Source: CAD feature listing. Evaluate the final solid. Frame: model axes, mm. Round coordinates to 2 decimals unless told otherwise and drop trailing zeros. Order: outer loops, then holes, each group sorted by start corner. A loop starts at its lowest first (then second) coordinate and runs counter-clockwise, first axis right, second up. Notation, with made-up numbers: M 14,83.25 L 61,83.25 A26 ccw 61,106.25 Z; hole C 9.25,-11 d7. An arc over 180 degrees is marked long. Answer as CSV lines item,"result". Start each with the question number.
Item 1: Section query B-B on y = 8. Return the cut outline in (x, z) (3 decimals).
Item 2: Line query: line 1 (Z direction, x = -53.5, y = 15) (3 decimals); line 2 (Z direction, x = -160.5, y = 18.5) (3 decimals); line 3 (Y direction, x = -162.5, z = 8) (3 decimals). Output: solid intervals per line, ascending. Write a range as [from, to].
Item 3: Section query A-A on x = -160.5. Return the cut outline in (y, z) (3 decimals), plus the area to 3 significant figures.
Item 4: First-contact query: P1, Ø1, axis at x = -78, z = 8.5, coming from the +Y side (3 decimals); P2, Ø5, axis at x = -209.5, y = 7.5, coming from the -Z side (3 decimals). Flat tips, straight axial feed; report the tip coordinate or a pass-through.
Item 5: Section query C-C on z = 5. Return the cut outline in (x, y) (3 decimals), plus the area to 3 significant figures.
from build123d import *

# Parameters (mm, degrees)
F0_W     = 19.05
F0_H     = 63.5
F1_DEPTH = 266.7
F2_SIZE2 = 15.875
F2_SIZE  = 15.875


with BuildPart() as f1:
    # F0 (on Right) → F1 (new body)
    with BuildSketch(Plane.YZ):
        with Locations((9.525, 31.75)):
            Rectangle(F0_W, F0_H)
    extrude(amount=-F1_DEPTH)

    # F2
    f2_edges = [f1.edges().sort_by_distance(p)[0] for p in [
        (-133.35, 19.05, 0),
    ]]
    chamfer(f2_edges, length=F2_SIZE, length2=F2_SIZE2)


solid = f1.part
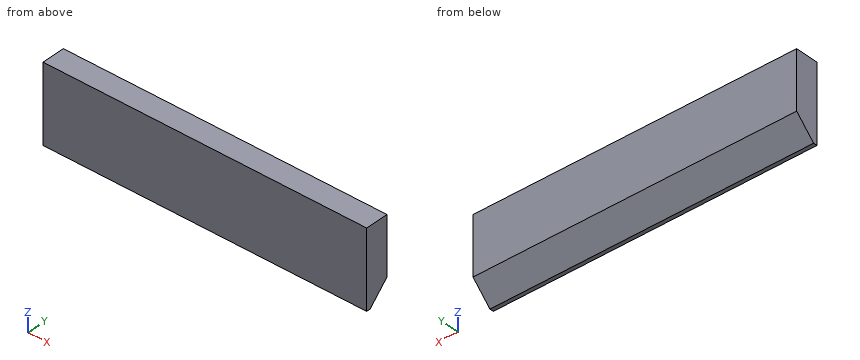
Results:
1,outline,"M -266.7,4.825 L 0,4.825 L 0,63.5 L -266.7,63.5 Z"
2,line 1,"[11.825, 63.5]"
2,line 2,"[15.325, 63.5]"
2,line 3,"[0, 11.175]"
3,outline,"M 0,0 L 3.175,0 L 19.05,15.875 L 19.05,63.5 L 0,63.5 Z"
3,area,"1,080 mm^2"
4,P1,"y = 12.175"
4,P2,"z = 1.825"
5,outline,"M -266.7,0 L 0,0 L 0,8.175 L -266.7,8.175 Z"
5,area,"2,180 mm^2"
